Geometry check sheet. Reference: the model listing, model coordinates, mm. Coordinates: 2 decimals unless noted, no trailing zeros. Write each loop counter-clockwise with the first axis right and the second up, starting at its lowest first coordinate (ties: lowest second). Pieces come first, ordered by that corner, then holes. Notation, with made-up numbers: (32.25, 81.25) -> (38.25, 81.25) arc R23 cw to (38.25, 102.25) -> close; hole circle Ø9 at (-7, 21.5). An arc over 180 degrees is marked (long way). Put each result on its own line as item: value. Start each with the question number.
from build123d import *

# Parameters (mm, degrees)
BOSS_EXTRUDE2_DEPTH = 1.8
FILLET1_R           = 5
CUT_EXTRUDE1_REACH  = 93.019
SKETCH3_R           = 1.6


with BuildPart() as part:
    # Sketch2 → Boss-Extrude2 (new body)
    with BuildSketch(Plane(origin=(0, 0, 0), x_dir=(1, 0, 0), z_dir=(0, 1, 0))):
        Polygon((-72.5, -55), (72.5, -55), (72.5, -42.3), (60.5, -42.3), (60.5, -8), (72.5, -8), (72.5, 8), (60.5, 8), (60.5, 42.3), (72.5, 42.3), (72.5, 55), (-72.5, 55), align=None)
    extrude(amount=BOSS_EXTRUDE2_DEPTH)

    # Fillet1
    fillet1_edges = [part.edges().sort_by_distance(p)[0] for p in [
        (72.5, 0.9, 55),
        (72.5, 0.9, -55),
    ]]
    fillet(fillet1_edges, radius=FILLET1_R)

    # Sketch3 → Cut-Extrude1 (cut, up to next)
    with BuildSketch(Plane(origin=(0, 1.8, 0), x_dir=(1, 0, 0), z_dir=(0, 1, 0)), mode=Mode.PRIVATE) as cut_extrude1_sk1:
        with Locations(Location((-68.8, 49.3, 0), (0, 0, 270))):
            Circle(SKETCH3_R)
    cut_extrude1_tool1 = extrude(cut_extrude1_sk1.sketch, amount=-CUT_EXTRUDE1_REACH, mode=Mode.PRIVATE) & part.part
    # Sketch3 → Cut-Extrude1 (cut, up to next)
    with BuildSketch(Plane(origin=(0, 1.8, 0), x_dir=(1, 0, 0), z_dir=(0, 1, 0)), mode=Mode.PRIVATE) as cut_extrude1_sk2:
        with Locations(Location((-1, 49.3, 0), (0, 0, 270))):
            Circle(SKETCH3_R)
    cut_extrude1_tool2 = extrude(cut_extrude1_sk2.sketch, amount=-CUT_EXTRUDE1_REACH, mode=Mode.PRIVATE) & part.part
    # Sketch3 → Cut-Extrude1 (cut, up to next)
    with BuildSketch(Plane(origin=(0, 1.8, 0), x_dir=(1, 0, 0), z_dir=(0, 1, 0)), mode=Mode.PRIVATE) as cut_extrude1_sk3:
        with Locations(Location((-1, -49.3, 0), (0, 0, 270))):
            Circle(SKETCH3_R)
    cut_extrude1_tool3 = extrude(cut_extrude1_sk3.sketch, amount=-CUT_EXTRUDE1_REACH, mode=Mode.PRIVATE) & part.part
    # Sketch3 → Cut-Extrude1 (cut, up to next)
    with BuildSketch(Plane(origin=(0, 1.8, 0), x_dir=(1, 0, 0), z_dir=(0, 1, 0)), mode=Mode.PRIVATE) as cut_extrude1_sk4:
        with Locations(Location((-68.8, -49.3, 0), (0, 0, 270))):
            Circle(SKETCH3_R)
    cut_extrude1_tool4 = extrude(cut_extrude1_sk4.sketch, amount=-CUT_EXTRUDE1_REACH, mode=Mode.PRIVATE) & part.part
    # Sketch3 → Cut-Extrude1 (cut, up to next)
    with BuildSketch(Plane(origin=(0, 1.8, 0), x_dir=(1, 0, 0), z_dir=(0, 1, 0)), mode=Mode.PRIVATE) as cut_extrude1_sk5:
        with Locations(Location((66.8, 49.3, 0), (0, 0, 270))):
            Circle(SKETCH3_R)
    cut_extrude1_tool5 = extrude(cut_extrude1_sk5.sketch, amount=-CUT_EXTRUDE1_REACH, mode=Mode.PRIVATE) & part.part
    # Sketch3 → Cut-Extrude1 (cut, up to next)
    with BuildSketch(Plane(origin=(0, 1.8, 0), x_dir=(1, 0, 0), z_dir=(0, 1, 0)), mode=Mode.PRIVATE) as cut_extrude1_sk6:
        with Locations(Location((66.8, -49.3, 0), (0, 0, 270))):
            Circle(SKETCH3_R)
    cut_extrude1_tool6 = extrude(cut_extrude1_sk6.sketch, amount=-CUT_EXTRUDE1_REACH, mode=Mode.PRIVATE) & part.part
    add(cut_extrude1_tool1.solids().sort_by_distance((-68.8, 1.8, -49.3))[0], mode=Mode.SUBTRACT)
    add(cut_extrude1_tool2.solids().sort_by_distance((-1, 1.8, -49.3))[0], mode=Mode.SUBTRACT)
    add(cut_extrude1_tool3.solids().sort_by_distance((-1, 1.8, 49.3))[0], mode=Mode.SUBTRACT)
    add(cut_extrude1_tool4.solids().sort_by_distance((-68.8, 1.8, 49.3))[0], mode=Mode.SUBTRACT)
    add(cut_extrude1_tool5.solids().sort_by_distance((66.8, 1.8, -49.3))[0], mode=Mode.SUBTRACT)
    add(cut_extrude1_tool6.solids().sort_by_distance((66.8, 1.8, 49.3))[0], mode=Mode.SUBTRACT)


solid = part.part
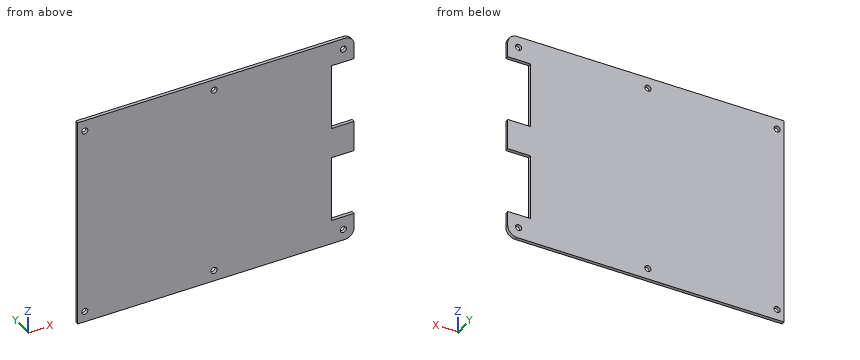
Item 1: Scan lines: line 1 along Z through (x, y) = (-68.8, 0.7); line 2 along X through (y, z) = (1.2, 49.3); line 3 along X through (y, z) = (1.7, -21.5). Record each from-to range of solid material in increasing order. Write a range as [from, to].
Item 2: Section check A-A, the plane x = -1. Enter the section's corners in (y, z), and give its area (3 significant figures).
Item 3: Section check B-B, the plane y = 0.75. Enter the section's corners in (x, z), and give its area (3 significant figures).
Item 4: Go/stop test with a flat-tipped pin: P1, Ø0.9, axis at y = 0.5, z = -17, coming from the +X side. Record where the tip stops, or that it passes through.
Item 5: Section check C-C, the plane z = -39.5. Enter the section's corners in (x, y).
From the geometry:
1. line 1: [-55, -50.9], [-47.7, 47.7], [50.9, 55]
1. line 2: [-72.5, -70.4], [-67.2, -2.6], [0.6, 65.2], [68.4, 72.5]
1. line 3: [-72.5, 60.5]
2. outline: (0, -55) -> (1.8, -55) -> (1.8, -50.9) -> (0, -50.9) -> close; (0, -47.7) -> (1.8, -47.7) -> (1.8, 47.7) -> (0, 47.7) -> close; (0, 50.9) -> (1.8, 50.9) -> (1.8, 55) -> (0, 55) -> close
2. area: 186 mm²
3. outline: (-72.5, -55) -> (67.5, -55) arc R5 ccw to (72.5, -50) -> (72.5, -42.3) -> (60.5, -42.3) -> (60.5, -8) -> (72.5, -8) -> (72.5, 8) -> (60.5, 8) -> (60.5, 42.3) -> (72.5, 42.3) -> (72.5, 50) arc R5 ccw to (67.5, 55) -> (-72.5, 55) -> close; hole circle Ø3.2 at (-68.8, -49.3); hole circle Ø3.2 at (-68.8, 49.3); hole circle Ø3.2 at (-1, -49.3); hole circle Ø3.2 at (-1, 49.3); hole circle Ø3.2 at (66.8, -49.3); hole circle Ø3.2 at (66.8, 49.3)
3. area: 15,100 mm²
4. P1: x = 60.5
5. outline: (-72.5, 0) -> (60.5, 0) -> (60.5, 1.8) -> (-72.5, 1.8) -> close
